Geometry: see drawing. Coordinates: mm, zero at the bounding-box minimum. Coordinates: 2 decimals unless noted, no trailing zeros. Write each loop counter-clockwise with the first axis right and the second up, starting at its lowest first coordinate (ties: lowest second). Pieces come first, ordered by that corner, then holes. Notation, with made-up numbers: (78, 62) -> (120, 62) arc R28 ccw to (120, 94) -> close; hole circle Ø11 at (14.25, -12). An arc over 180 degrees is marked (long way). Answer as a JSON object with one key per item and string values. Group by question number.
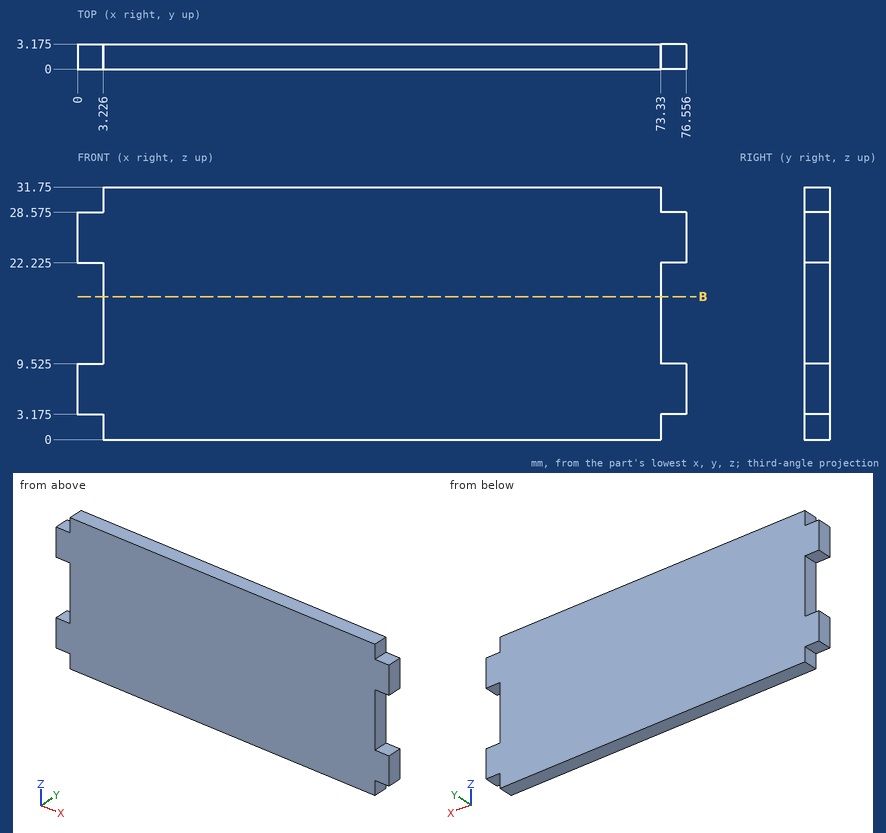
Item 1: Contact query for flat-ended pins moving along their axis: pin 1 (1 mm diameter, centred on y = 2, z = 29.5, fed in from -X); pin 2 (1.6 mm diameter, centred on y = 1, z = 16, fed in from +X); pin 3 (1.6 mm diameter, centred on x = 75, y = 1, fed in from +Z) (3 decimals). Output: stop coordinate, or through.
Item 2: Section B-B on z = 18. Output: boundary loops of the cut face in (x, y) (1 decimal).
Item 3: Ray query, L1, parallel to X at y = 1.6, z = 14.5 (1 decimal). Return the intervals inside material, ascending. Write a range as [from, to].
Answer sheet:
{
 "1": {"pin 1": "stops at x = 3.23", "pin 2": "stops at x = 73.33", "pin 3": "stops at z = 28.575"},
 "2": {"outline": "(3.2, 0) -> (73.3, 0) -> (73.3, 3.2) -> (3.2, 3.2) -> close"},
 "3": {"L1": "x = [3.2, 73.3]"}
}
